Autodesk Fusion 360 part; units mm, degrees
sketch "Sketch1" plane through (0, 0, 0) normal (0, 0, 1) x (1, 0, 0)
  circle A0 centre (0, 0) radius 22.5
  circle A1 centre (10.9935, 0) radius 15
  line L0 (21.0297, 6) -> (24.7412, 6)
  line L1 (21.3005, -6) -> (24.7412, -6)
  line L2 (-24.0211, 0.3833) -> (-31.0114, 0.3928) construction
  line L3 (0, 0) -> (31, 0) construction
  dimension "d2" = 45
  dimension "d3" = 30
  dimension "d6" = 6
  dimension "d7" = 6
extrude "Extrude1" add sketch "Sketch1" along normal blind 90 contours A0 A1 L0 L1
ref_plane "WorkPlane1" through (25.9935, 0, 55.0321) normal (1, 0, 0) x (0, -1, 0)
sketch "Sketch2" plane through (25.9935, 0, 0) normal (1, 0, 0) x (0, 1, 0)
  circle A0 centre (0, 75) radius 1.7
  circle A1 centre (0, 15) radius 1.7
  line L0 (6, 90) -> (-6, 90)
  dimension "d11" = 60
  dimension "d12" = 3.4
  dimension "d15" = 15
extrude "Extrude2" cut sketch "Sketch2" against normal blind 25
ref_plane "WorkPlane2" through (25.9935, 0, 73.0088) normal (1, 0, 0) x (0, -1, 0)
sketch "Sketch3" plane through (25.9935, 0, 0) normal (1, 0, 0) x (0, 1, 0)
  line L0 (-6, 90) -> (6, 90)
  line L1 (6, 90) -> (6, 0)
  line L2 (6, 0) -> (-6, 0)
  line L3 (-6, 0) -> (-6, 90)
  line L4 (0, 0) -> (0, 98.2362) construction
  dimension "d22" = 12
  dimension "d23" = 6
extrude "Extrude3" cut sketch "Sketch3" against normal blind 1.5
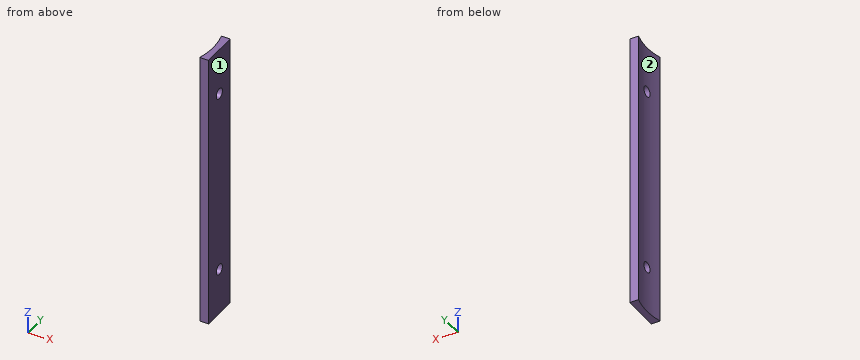
Verification items for the finished model (mm, model axes). Face numbers are marked on the shaded views. Give positions to 0.01 mm unless a question says otherwise; leave off trailing zeros. Order: outer loops, then holes, each group sorted by start corner. A loop starts at its lowest first (then second) coordinate and runs counter-clockwise, first axis right, second up. Notation, with made-up numbers: (-19.5, 24) -> (-15.5, 24) arc R23 ccw to (-15.5, 40) -> close; hole circle Ø9 at (73, -35.75). An arc over 180 degrees is marked (long way). Use a Markdown table: item, result.
1) Section check C-C, the plane x = 24.05. Record the boundary of the cut face in (y, z).
Results:
| item | result |
|---|---|
| outline | (-6, 0) -> (6, 0) -> (6, 90) -> (-6, 90) -> close; hole circle Ø3.4 at (0, 15); hole circle Ø3.4 at (0, 75) |
2) Section check B-B, the plane y = 0. Record the boundary of the cut face in (x, z), then the cut area to 3 significant figures.
Results:
| item | result |
|---|---|
| outline | (22.5, 0) -> (24.49, 0) -> (24.49, 13.3) -> (22.5, 13.3) -> close; (22.5, 16.7) -> (24.49, 16.7) -> (24.49, 73.3) -> (22.5, 73.3) -> close; (22.5, 76.7) -> (24.49, 76.7) -> (24.49, 90) -> (22.5, 90) -> close |
| area | 166 mm² |
3) Material ranges on probe 1 along Z at (x, y) = (23.25, 0); probe 2 along Z at (x, y) = (22.8, -0.5); probe 3 along X at (y, z) = (0.75, 73), recorded low to high.
Results:
| item | result |
|---|---|
| probe 1 | 0 to 13.3, 16.7 to 73.3, 76.7 to 90 |
| probe 2 | 0 to 13.38, 16.62 to 73.38, 76.62 to 90 |
| probe 3 | 22.49 to 24.49 |
4) Mould release check, pull along Y, two halves, no side actions. Record for the marked faces 1 and 2: pulls with the +Y half, pulls with the -Y half, needs draft (parallel to the pull), parting line crosses it, or undercut.
Results:
| item | result |
|---|---|
| face 1 | needs draft |
| face 2 | undercut |
5) Section check D-D, the plane z = 58. Record the boundary of the cut face in (x, y), then the cut area to 3 significant figures.
Results:
| item | result |
|---|---|
| outline | (21.69, -6) -> (24.49, -6) -> (24.49, 6) -> (21.69, 6) arc R22.5 cw to start |
| area | 27.2 mm² |
6) Section check A-A, the plane z = 75. Record the boundary of the cut face in (x, y), then the cut area to 3 significant figures.
Results:
| item | result |
|---|---|
| outline | (21.69, -6) -> (24.49, -6) -> (24.49, -1.7) -> (22.44, -1.7) arc R22.5 cw to start; (21.69, 6) arc R22.5 cw to (22.44, 1.7) -> (24.49, 1.7) -> (24.49, 6) -> close |
| area | 20.3 mm² |
7) Depth check by flat-ended pin: pin 1 Ø1.5 at (y, z) = (2, 65.5) entering from -X; pin 2 Ø5.5 at (y, z) = (0, 15) entering from +X; pin 3 Ø1.5 at (y, z) = (3.5, 70) entering from -X; pin 4 Ø3 at (y, z) = (3.5, 28) entering from -X. Enter the tip coordinate at first touch or a pass-through.
Results:
| item | result |
|---|---|
| pin 1 | x = 22.33 |
| pin 2 | x = 24.49 |
| pin 3 | x = 22.09 |
| pin 4 | x = 21.94 |
